from build123d import *

# Parameters (mm, degrees)
BOX002_W     = 275
BOX002_H     = 275
BOX002_DEPTH = 47
SKETCH022_W  = 195
SKETCH022_H  = 195
SKETCH023_W  = 180
SKETCH023_H  = 180
BOX001_W     = 275
BOX001_H     = 275
BOX001_DEPTH = 52
SKETCH020_W  = 275
SKETCH020_H  = 275
SKETCH021_W  = 0.1
SKETCH021_H  = 0.1
SKETCH018_W  = 275
SKETCH018_H  = 275
SKETCH019_W  = 0.1
SKETCH019_H  = 0.1
BOX_W        = 275
BOX_H        = 275
BOX_DEPTH    = 57


with BuildPart() as layer0keep001:
    # Box002 → Box002 (new body)
    with BuildSketch(Plane.XY):
        with Locations((137.5, 137.5)):
            Rectangle(BOX002_W, BOX002_H)
    extrude(amount=BOX002_DEPTH)


with BuildPart() as layer003:
    # Sketch022 → Loft003 section 0
    with BuildSketch(Plane.XY.offset(47)):
        with Locations((137.5, 137.5)):
            Rectangle(SKETCH022_W, SKETCH022_H)
    # Sketch023 → Loft003 section 1
    with BuildSketch(Plane.XY.offset(57)):
        with Locations((137.5, 137.5)):
            Rectangle(SKETCH023_W, SKETCH023_H)
    loft()

    # Fusion015: union layer0Keep001
    add(layer0keep001.part)


with BuildPart() as layer002:
    # Box001 → Box001 (new body)
    with BuildSketch(Plane.XY.offset(5)):
        with Locations((137.5, 137.5)):
            Rectangle(BOX001_W, BOX001_H)
    extrude(amount=BOX001_DEPTH)


with BuildPart() as layer0cut:
    # Sketch020 → Loft002 section 0
    with BuildSketch(Plane.XY):
        with Locations((137.5, 137.5)):
            Rectangle(SKETCH020_W, SKETCH020_H)
    # Sketch021 → Loft002 section 1
    with BuildSketch(Plane.XY.offset(175.1)):
        with Locations((137.5, 137.5)):
            Rectangle(SKETCH021_W, SKETCH021_H)
    loft()


with BuildPart() as layer0cut_1:
    # Loft002 placement: moved
    add(layer0cut.part.moved(Location((0, 0, -6))))

    # Common001: intersect layer002
    add(layer002.part, mode=Mode.INTERSECT)


with BuildPart() as obj1:
    # Sketch018 → Loft001 section 0
    with BuildSketch(Plane.XY):
        with Locations((137.5, 137.5)):
            Rectangle(SKETCH018_W, SKETCH018_H)
    # Sketch019 → Loft001 section 1
    with BuildSketch(Plane.XY.offset(175.1)):
        with Locations((137.5, 137.5)):
            Rectangle(SKETCH019_W, SKETCH019_H)
    loft()


with BuildPart() as obj2:
    # Box → Box (new body)
    with BuildSketch(Plane.XY):
        with Locations((137.5, 137.5)):
            Rectangle(BOX_W, BOX_H)
    extrude(amount=BOX_DEPTH)

    # Common: intersect obj1
    add(obj1.part, mode=Mode.INTERSECT)

    # Cut: cut layer0cut
    add(layer0cut_1.part, mode=Mode.SUBTRACT)

    # Common002: intersect layer003
    add(layer003.part, mode=Mode.INTERSECT)


solid = obj2.part
For this review, take the finished solid that the model builds, in its own axes (mm). Round coordinates to 2 decimals unless told otherwise and drop trailing zeros. Put each result on its own line as item: value. Start each with the question number.
1. For probe 1 along Z at (x, y) = (102.5, 89); probe 2 along Y at (x, z) = (32, 30.5); probe 3 along Z at (x, y) = (248, 62), list the stretches that pass through material, from the lowest coordinate up. Write a range as [from, to].
2. Insertion check: P1, Ø5, axis at y = 95.5, z = 28, coming from the -X side; P2, Ø8, axis at x = 213.5, y = 68.5, coming from the +Z side; P3, Ø12, axis at y = 98, z = 26, coming from the +X side. Each pin has a flat end and moves straight along its axis. Give the tip position at first contact, or say it passes through.
3. Mouldability with a two-part tool opening along Z and no side actions: class faces 1 (the flat face through (136, 139, 5)), 2 (the flat face through (136, 139, 0)) as +Z half, -Z half, draft (parallel to the pull), parting line (faces both ways), or undercut.
Result sheet:
1. probe 1: [0, 5]
1. probe 2: [23.94, 28.65], [246.35, 251.06]
1. probe 3: [0, 5], [28.4, 34.4]
2. P1: x = 20.02
2. P2: z = 5
2. P3: x = 259.3
3. face 1: undercut
3. face 2: -Z half
